from build123d import *

# Parameters (mm, degrees)
F2_DEPTH  = 140
F3_DEPTH  = 25.4
F6_W      = 215.1558175683
F6_H      = 84.3175165355
F7_DEPTH  = 140.001
F9_DEPTH  = 140.001
F5_R      = 15.5218481215
F10_DEPTH = 44.4123579555
F10_TAPER = -3


with BuildPart() as f2:
    # F1 (on offset) → F2 (new body)
    with BuildSketch(Plane.YZ.offset(-70)):
        with BuildLine():
            Line((0, 67.9838731885), (0, 0))
            Line((0, 0), (19.0113577992, 0))
            ThreePointArc((19.0113577992, 0), (14.1699092565, 35.2962658126), (0, 67.9838731885))
        make_face()
        with BuildLine():
            Line((19.0113577992, 0), (0, 0))
            Line((0, 0), (0, -67.971073091))
            ThreePointArc((0, -67.971073091), (14.1681854898, -35.2896292573), (19.0113577992, 0))
        make_face()
    extrude(amount=F2_DEPTH)

    # F3 (add): a face of the model
    f3_faces = [f2.faces().sort_by_distance(p)[0] for p in [
        (0, 0, 0.0064000487),
    ]]
    extrude(f3_faces, amount=F3_DEPTH)

    # F6 (on offset) → F7 (cut, through all)
    with BuildSketch(Plane.YZ.offset(-70)):
        with Locations((27.4681784213, 72.3114386201)):
            Rectangle(F6_W, F6_H)
    extrude(amount=F7_DEPTH, mode=Mode.SUBTRACT)

    # F8 (on face) → F9 (cut, through all)
    with BuildSketch(Plane(origin=(-70, 0, 0), x_dir=(0, -1, 0), z_dir=(-1, 0, 0))):
        Polygon((0, -67.971073091), (25.4, -67.971073091), (25.4, -42.571246624), align=None)
    extrude(amount=-F9_DEPTH, mode=Mode.SUBTRACT)

    # F5 (on face) → F10 (cut, through all)
    with BuildSketch(Plane.XZ.offset(25.4)):
        with Locations((-35.0152216852, 0)):
            Circle(F5_R)
        with BuildLine():
            ThreePointArc((50.4853369025, 0), (35.0099764764, 15.4753604261), (19.5346160504, 0))
            ThreePointArc((19.5346160504, 0), (35.0099764764, -15.4753604261), (50.4853369025, 0))
        make_face()
    extrude(amount=-F10_DEPTH, taper=F10_TAPER, mode=Mode.SUBTRACT)


solid = f2.part
Can you work these out from the model? Positions are in its coordinate system, mm. Round coordinates to 2 decimals unless told otherwise and drop trailing zeros. Order: outer loops, then holes, each group sorted by start corner. A loop starts at its lowest first (then second) coordinate and runs counter-clockwise, first axis right, second up. Notation, with made-up numbers: M 42,39 L 77,39 A15 ccw 77,68 Z; hole C -1,-13 d9. An arc over 180 degrees is marked long. Use a Markdown table: item, result.
1) Imagine slicing it at C-C (z = -7). Give the number of separate pieces and of enclosed holes in the cut face, then the cut area to 3 significant figures.
Geometry says:
| item | result |
|---|---|
| separate pieces | 3 |
| enclosed holes | 0 |
| area | 3,520 mm² |
2) Imagine slicing it at A-A (y = 5.5). List the corners of the cut face in (x, z) for me, then the cut area to 3 significant figures.
Geometry says:
| item | result |
|---|---|
| outline | M -70,-57.95 L 70,-57.95 L 70,30.15 L -70,30.15 Z; hole C -35.02,0 d34.28; hole C 35.01,0 d34.19 |
| area | 10,500 mm² |
3) I'm going to push flat-ended pins straight in: P1, Ø8, axis at x = -44, y = 10, coming from the -Z side; P2, Ø5, axis at x = 7.5, z = -3.5, coming from the +Y side; P3, Ø6, axis at x = 36.5, y = -11.5, coming from the -Z side. Where does each tip first touch, or does it pass through?
Geometry says:
| item | result |
|---|---|
| P1 | stops at z = -56.92 |
| P2 | stops at y = 19.01 |
| P3 | stops at z = -59.47 |
4) If I drill on line 1 along X through (y, z) = (7.5, -5); line 2 along X through (y, z) = (15, -12); line 3 along Z through (x, y) = (48, -7), over which ranges is the centre line in solid material (lowest first)?
Geometry says:
| item | result |
|---|---|
| line 1 | x = -70 to -51.52, -18.51 to 18.55, 51.47 to 70 |
| line 2 | x = -70 to -47.94, -22.09 to 22.15, 47.87 to 70 |
| line 3 | z = -60.97 to -10.08, 10.08 to 30.15 |
5) If we mould it in two halves opening along X, with no side actions, what happens to faces 1 (the face through (70, -3, -7)), 2 (the face through (-38.636, -2.883, -16.305)), 3 (the face through (-70, -3, -7)), 4 (the face through (-1, -5, 30.153))? For each: +X half, -X half, draft (parallel to the pull), parting line (faces both ways), or undercut.
Geometry says:
| item | result |
|---|---|
| face 1 | +X half |
| face 2 | undercut |
| face 3 | -X half |
| face 4 | draft |
6) Imagine slicing it at D-D (y = -16). List the corners of the cut face in (x, z) for me, then the cut area to 3 significant figures.
Geometry says:
| item | result |
|---|---|
| outline | M -70,-51.97 L 70,-51.97 L 70,30.15 L -70,30.15 Z; hole C -35.02,0 d32.03; hole C 35.01,0 d31.94 |
| area | 9,890 mm² |
7) Imagine slicing it at B-B (x = -4). List the corners of the cut face in (y, z) for me, then the cut area to 3 significant figures.
Geometry says:
| item | result |
|---|---|
| outline | M -25.4,-42.57 L 0,-67.97 A131.04 ccw 15.5,30.15 L -25.4,30.15 Z |
| area | 3,580 mm² |
